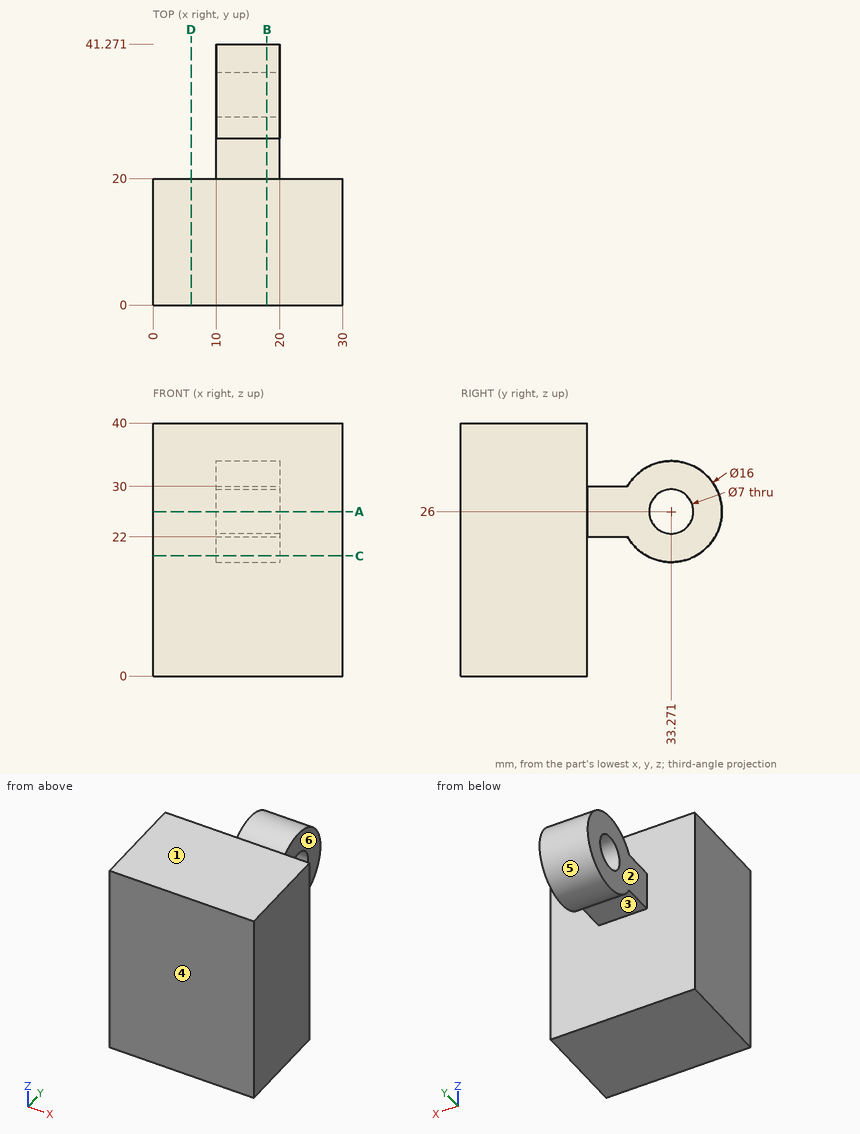
Design review of the part shown in the three views and the two pictorial views. Dimensions are in mm from the part's minimum x, y and z. A direction names the side the tool comes from. Round coordinates to 2 decimals unless told otherwise and drop trailing zeros. Write each loop counter-clockwise with the first axis right and the second up, starting at its lowest first coordinate (ties: lowest second). Pieces come first, ordered by that corner, then holes.
Item 1: For the marked faces 1 and 2, list the 3-axis set-ups (+Z, -Z, +X, -X, +Y, -Y) from which the entire face can be reached by the end or side of a thin tool; tool diameter is ignored.
Item 2: The part is to be moulded in two halves that separate along Y. For the marked faces 3, 4, 5 and 6, say which applies: +Y half, -Y half, draft (parallel to the pull), parting line (faces both ways), or undercut.
Item 3: We need section A-A on z = 26. Write out the cut boundary in (x, y).
Item 4: We need section C-C on z = 19. Write out the cut boundary in (x, y), and give its area (3 significant figures).
Item 5: Clearance check with flat-ended pins moving along their axes: pin 1 Ø17.5 at (y, z) = (26.5, 25) entering from -X; pin 2 Ø5.5 at (y, z) = (33.27, 26) entering from -X; pin 3 Ø13 at (y, z) = (29.5, 23.5) entering from +X; pin 4 Ø1.9 at (x, y) = (16.5, 24) entering from -Z. State where each tip first meets the part, or that it passes through.
Item 6: For probe 1 along Y at (x, z) = (18.25, 26); probe 2 along Y at (x, z) = (24.75, 21); probe 3 along X at (y, z) = (36, 19), list the stretches that pass through material, from the lowest coordinate up.
Item 7: We need section B-B on x = 18. Write out the cut boundary in (y, z), and give its area (3 significant figures).
Item 8: We need section D-D on x = 6. Write out the cut boundary in (y, z), and give its area (3 significant figures).
Returned:
1. face 1: +Z, +X, -X, +Y, -Y
1. face 2: +Z, -Z, -X, +Y
2. face 3: undercut
2. face 4: -Y half
2. face 5: undercut
2. face 6: draft
3. outline: (0, 0) - (30, 0) - (30, 20) - (20, 20) - (20, 29.77) - (10, 29.77) - (10, 20) - (0, 20) - close; (10, 36.77) - (20, 36.77) - (20, 41.27) - (10, 41.27) - close
4. outline: (0, 0) - (30, 0) - (30, 20) - (0, 20) - close; (10, 29.4) - (20, 29.4) - (20, 37.14) - (10, 37.14) - close
4. area: 677 mm2
5. pin 1: stops at x = 0
5. pin 2: passes through
5. pin 3: stops at x = 20
5. pin 4: stops at z = 22
6. probe 1: y = 0 to 29.77, 36.77 to 41.27
6. probe 2: y = 0 to 20
6. probe 3: x = 10 to 20
7. outline: (0, 0) - (20, 0) - (20, 22) - (26.34, 22) arc R8 ccw (long way) to (26.34, 30) - (20, 30) - (20, 40) - (0, 40) - close; hole circle Ø7 at (33.27, 26)
7. area: 1,010 mm2
8. outline: (0, 0) - (20, 0) - (20, 40) - (0, 40) - close
8. area: 800 mm2
